```python
from build123d import *

# Parameters (mm, degrees)
SKETCH_1_W          = 20
SKETCH_1_H          = 140
SKETCH_1_R          = 2.25
EXTRUDE_1_DEPTH     = 12
FILLET_1_R          = 20
SKETCH_2_W          = 19.364916731
SKETCH_2_H          = 15
CUT_EXTRUDE_1_DEPTH = 72.721684308


with BuildPart() as part:
    # 草图1 → 凸台-拉伸1 (new body)
    with BuildSketch(Plane.XY):
        Rectangle(SKETCH_1_W, SKETCH_1_H)
        with Locations((0, -50)):
            Circle(SKETCH_1_R, mode=Mode.SUBTRACT)
        Circle(SKETCH_1_R, mode=Mode.SUBTRACT)
        with Locations((0, 50)):
            Circle(SKETCH_1_R, mode=Mode.SUBTRACT)
    extrude(amount=EXTRUDE_1_DEPTH)

    # 圆角1
    fillet_1_edges = [part.edges().sort_by_distance(p)[0] for p in [
        (10, -70, 6),
        (10, 70, 6),
    ]]
    fillet(fillet_1_edges, radius=FILLET_1_R - 0.0001)  # a hair under: the kernel refuses the full size

    # 草图2 → 切除-拉伸1 (cut, through all)
    with BuildSketch(Plane.XY.offset(12)):
        with Locations((-0.317541634, 62.5)):
            Rectangle(SKETCH_2_W, SKETCH_2_H)
    extrude(amount=-CUT_EXTRUDE_1_DEPTH, mode=Mode.SUBTRACT)


solid = part.part
```
The listing builds one solid part. Answer for the finished solid, in the listing's coordinates (mm). Round coordinates to 2 decimals unless told otherwise and drop trailing zeros. Loops run counter-clockwise (first coordinate to the right, second up) from the corner with the lowest first, then second, coordinate; pieces in that order, holes last. Notation, with made-up numbers: (-27.75, 79) - (31.25, 79) arc R12 cw to (31.25, 97) - close; hole circle Ø7 at (12.25, 30). An arc over 180 degrees is marked (long way). Return JSON: item names as keys, results as strings. Group by question number.
1. Consider probe 1 along Y at (x, z) = (0, 4.75); probe 2 along Y at (x, z) = (-1, 8.5); probe 3 along Y at (x, z) = (-8.5, 2.5). Determine where each line is inside the solid, lowest interval first.
2. The part is cut by section A-A on y = 0. Determine the outline of the cut face in (x, z).
3. The mould has two halves that part along X. Classify faces 1 (the cylindrical face through (-0.29, 52.23, 5.92)), 2 (the flat face through (0, -7, 0)), 3 (the flat face through (-10, -8, 6)): pulls with the +X half, pulls with the -X half, needs draft (parallel to the pull), parting line crosses it, or undercut.
4. The part is cut by section C-C on z = 5. State how many separate pieces and enclosed holes the cut face has, then the cut area to 3 significant figures.
5. The part is cut by section B-B on x = 0. Determine the outline of the cut face in (y, z).
6. Each of these flat-tipped pins is pushed along its axis until it touches: P1, Ø2.5, axis at x = 0, y = 0, coming from the -Z side; P2, Ø1.5, axis at x = -4.5, z = 10.5, coming from the -Y side. Where does it stop, or does it pass through?
Resolved:
{
 "1": {"probe 1": "y = -67.32 to -52.25, -47.75 to -2.25, 2.25 to 47.75, 52.25 to 55", "probe 2": "y = -67.86 to -52.02, -47.98 to -2.02, 2.02 to 47.98, 52.02 to 55", "probe 3": "y = -69.94 to 55"},
 "2": {"outline": "(-10, 0) - (-2.25, 0) - (-2.25, 12) - (-10, 12) - close; (2.25, 0) - (10, 0) - (10, 12) - (2.25, 12) - close"},
 "3": {"face 1": "undercut", "face 2": "needs draft", "face 3": "pulls with the -X half"},
 "4": {"separate pieces": "1", "enclosed holes": "3", "area": "2,370 mm²"},
 "5": {"outline": "(-67.32, 0) - (-52.25, 0) - (-52.25, 12) - (-67.32, 12) - close; (-47.75, 0) - (-2.25, 0) - (-2.25, 12) - (-47.75, 12) - close; (2.25, 0) - (47.75, 0) - (47.75, 12) - (2.25, 12) - close; (52.25, 0) - (55, 0) - (55, 12) - (52.25, 12) - close"},
 "6": {"P1": "passes through", "P2": "stops at y = -69.43"}
}
